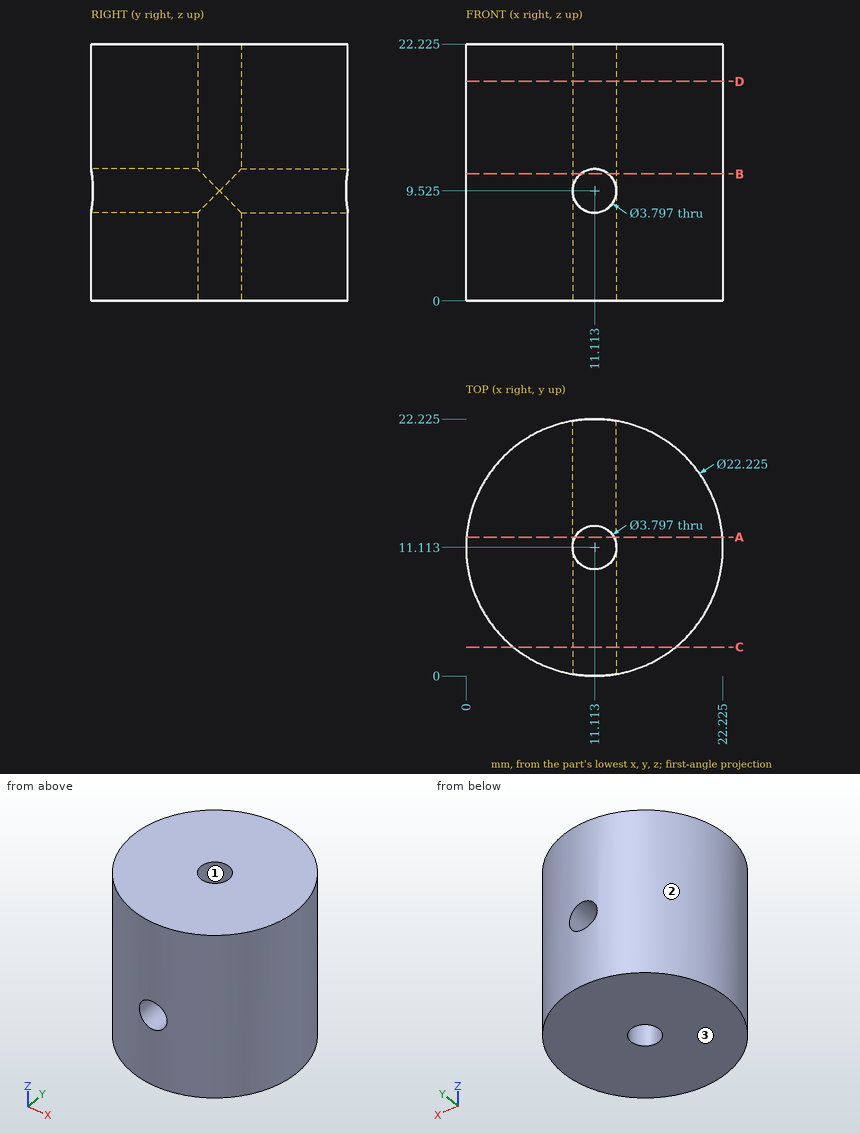
Check sheet for the drawn part. Datum: minimum x, y, z corner. Units: mm. Coordinates: 2 decimals unless noted, no trailing zeros. Order: outer loops, then holes, each group sorted by start corner. A loop starts at its lowest first (then second) coordinate and runs counter-clockwise, first axis right, second up. Notation, with made-up numbers: M -34.75,4.25 L 0.25,4.25 A27 cw 0.25,32.25 Z; hole C 88.25,3 d11. An arc over 180 degrees is marked long. One line per item, written item: value. Start each with the question number.
Item 1: Mould release check, pull along X, two halves, no side actions. Record for the marked faces 1, 2 and 3: released by +X, released by -X, zero draft, split by the parting line, or undercut.
Item 2: Sectioned sample at B-B (z = 11). Enter the section's corners in (x, y) (1 decimal).
Item 3: Sectioned sample at A-A (y = 12). Enter the section's corners in (x, z) (1 decimal), then the cut area to 3 significant figures.
Item 4: Gauge pin test, flat ends, axial feed: pin 1 (1.5 mm diameter, centred on y = 3.5, z = 6, fed in from +X); pin 2 (8 mm diameter, centred on y = 5.5, z = 17.5, fed in from +X); pin 3 (5 mm diameter, centred on x = 11.11, z = 9.53, fed in from -Y); pin 4 (8 mm diameter, centred on y = 4, z = 13.5, fed in from +X). Record the tip position at first contact, or that the pin passes through.
Item 5: Sectioned sample at C-C (y = 2.5). Enter the section's corners in (x, z) (1 decimal).
Item 6: Scan lines: probe 1 along X at (y, z) = (11, 17) (1 decimal); probe 2 along X at (y, z) = (17.5, 9.5) (1 decimal); probe 3 along Y at (x, z) = (10.25, 6.75) (1 decimal). Record each from-to range of solid material in increasing order.
Item 7: Sectioned sample at D-D (z = 19). Enter the section's corners in (x, y) (1 decimal), then the cut area to 3 significant figures.
Conclusion:
1. face 1: undercut
1. face 2: split by the parting line
1. face 3: zero draft
2. outline: M 9.9,0.1 L 9.9,9.6 A1.9 cw 9.9,12.6 L 9.9,22.2 A11.1 ccw Z; M 12.3,0.1 A11.1 ccw 12.3,22.2 L 12.3,12.6 A1.9 cw 12.3,9.6 Z
3. outline: M 0,0 L 9.4,0 L 9.4,8.6 A1.9 cw 9.4,10.4 L 9.4,22.2 L 0,22.2 Z; M 12.8,0 L 22.2,0 L 22.2,22.2 L 12.8,22.2 L 12.8,10.4 A1.9 cw 12.8,8.6 Z
3. area: 417 mm^2
4. pin 1: stops at x = 19.85
4. pin 2: stops at x = 22.11
4. pin 3: stops at y = 0
4. pin 4: stops at x = 21.78
5. outline: M 4.1,0 L 18.1,0 L 18.1,22.2 L 4.1,22.2 Z; hole C 11.1,9.5 d3.8
6. probe 1: x = 0 to 9.2, 13 to 22.2
6. probe 2: x = 2 to 9.2, 13 to 20.2
6. probe 3: y = 0 to 9.4, 12.8 to 22.2
7. outline: C 11.1,11.1 d22.2; hole C 11.1,11.1 d3.8
7. area: 377 mm^2
